Can you work these out from the model? Positions are in its coordinate system, mm. A direction names the side the tool comes from. Give positions to 0.01 mm unless a question says otherwise; leave off trailing zeros. Order: outer loops, then holes, each group sorted by start corner. A loop starts at its lowest first (then second) coordinate and runs counter-clockwise, first axis right, second up. Notation, with made-up numbers: (82, 73.25) - (99, 73.25) arc R32 ccw to (99, 110.25) - close; hole circle Ø10 at (-0.5, 81.25). An arc over 180 degrees is marked (long way). Answer as a JSON object with one key per item and string values.
```python
from build123d import *

# Parameters (mm, degrees)
SKETCH1_R           = 3.95
SKETCH1_R_2         = 1.475
SKETCH1_R_3         = 22.5
SKETCH1_R_4         = 2.4
SKETCH1_R_5         = 1.975
BOSS_EXTRUDE1_DEPTH = 5


with BuildPart() as part:
    # Sketch1 → Boss-Extrude1 (new body)
    with BuildSketch(Plane.XY):
        with BuildLine():
            Line((35, 0), (35, 162))
            ThreePointArc((35, 162), (0, 197), (-35, 162))
            Line((-35, 162), (-35, 0))
            ThreePointArc((-35, 0), (0, -35), (35, 0))
        make_face()
        Circle(SKETCH1_R, mode=Mode.SUBTRACT)
        with Locations((0, 29)):
            Circle(SKETCH1_R_2, mode=Mode.SUBTRACT)
        with Locations((0, 162)):
            Circle(SKETCH1_R_3, mode=Mode.SUBTRACT)
        with Locations((0, 133)):
            Circle(SKETCH1_R_2, mode=Mode.SUBTRACT)
        with Locations((-30, 97)):
            Circle(SKETCH1_R_2, mode=Mode.SUBTRACT)
        with Locations((30, 97)):
            Circle(SKETCH1_R_2, mode=Mode.SUBTRACT)
        with Locations((29, 0)):
            Circle(SKETCH1_R_2, mode=Mode.SUBTRACT)
        with Locations((0, -29)):
            Circle(SKETCH1_R_2, mode=Mode.SUBTRACT)
        with Locations((-29, 0)):
            Circle(SKETCH1_R_2, mode=Mode.SUBTRACT)
        with Locations((0, 12)):
            Circle(SKETCH1_R_4, mode=Mode.SUBTRACT)
        with Locations((12, 0)):
            Circle(SKETCH1_R_4, mode=Mode.SUBTRACT)
        with Locations((0, -12)):
            Circle(SKETCH1_R_4, mode=Mode.SUBTRACT)
        with Locations((-12, 0)):
            Circle(SKETCH1_R_4, mode=Mode.SUBTRACT)
        with Locations((0, 191)):
            Circle(SKETCH1_R_5, mode=Mode.SUBTRACT)
        with Locations((29, 162)):
            Circle(SKETCH1_R_5, mode=Mode.SUBTRACT)
        with Locations((-29, 162)):
            Circle(SKETCH1_R_5, mode=Mode.SUBTRACT)
        with BuildLine():
            Line((4.5, 80), (4.5, 40))
            ThreePointArc((4.5, 40), (0, 35.5), (-4.5, 40))
            Line((-4.5, 40), (-4.5, 80))
            ThreePointArc((-4.5, 80), (0, 84.5), (4.5, 80))
        make_face(mode=Mode.SUBTRACT)
        with BuildLine():
            Line((21.5, 80), (21.5, 40))
            ThreePointArc((21.5, 40), (17, 35.5), (12.5, 40))
            Line((12.5, 40), (12.5, 80))
            ThreePointArc((12.5, 80), (17, 84.5), (21.5, 80))
        make_face(mode=Mode.SUBTRACT)
        with BuildLine():
            Line((-21.5, 80), (-21.5, 40))
            ThreePointArc((-21.5, 40), (-17, 35.5), (-12.5, 40))
            Line((-12.5, 40), (-12.5, 80))
            ThreePointArc((-12.5, 80), (-17, 84.5), (-21.5, 80))
        make_face(mode=Mode.SUBTRACT)
        with BuildLine():
            Line((6.5, 121.5), (6.5, 108.5))
            ThreePointArc((6.5, 108.5), (0, 102), (-6.5, 108.5))
            Line((-6.5, 108.5), (-6.5, 121.5))
            ThreePointArc((-6.5, 121.5), (0, 128), (6.5, 121.5))
        make_face(mode=Mode.SUBTRACT)
        with BuildLine():
            Line((26.5, 120.946496324), (26.5, 107.946496324))
            ThreePointArc((26.5, 107.946496324), (20, 101.446496324), (13.5, 107.946496324))
            Line((13.5, 107.946496324), (13.5, 120.946496324))
            ThreePointArc((13.5, 120.946496324), (20, 127.446496324), (26.5, 120.946496324))
        make_face(mode=Mode.SUBTRACT)
        with BuildLine():
            Line((-26.5, 120.946496324), (-26.5, 107.946496324))
            ThreePointArc((-26.5, 107.946496324), (-20, 101.446496324), (-13.5, 107.946496324))
            Line((-13.5, 107.946496324), (-13.5, 120.946496324))
            ThreePointArc((-13.5, 120.946496324), (-20, 127.446496324), (-26.5, 120.946496324))
        make_face(mode=Mode.SUBTRACT)
    extrude(amount=BOSS_EXTRUDE1_DEPTH)


solid = part.part
```
Q1. We'd pull the mould along X, two halves only. Please class faces 1 (the face through (0.77, 196.99, 2.46)), 2 (the face through (0.1, 35.5, 2.5)), 3 (the face through (-19.857, 127.445, 2.465)), 4 (the face through (7, 83, 5)): released by +X, released by -X, zero draft, split by the parting line, or undercut.
Recorded:
{"face 1": "split by the parting line", "face 2": "undercut", "face 3": "undercut", "face 4": "zero draft"}
Q2. Which directions (+Z, -Z, +X, -X, +Y, -Y) give clear straight access to the entire face, cutting with the end or side of a thin tool? Please do faces 5 (the face through (0, 128, 2)), 6 (the face through (35, 80, 2)).
Recorded:
{"face 5": "+Z, -Z", "face 6": "+Z, -Z, +X, +Y, -Y"}
Q3. If we section it at B-B, the plane y = 146.5: Please give me the cut outline in (x, z), then the cut area to 3 significant figures.
Recorded:
{"outline": "(-35, 0) - (-16.31, 0) - (-16.31, 5) - (-35, 5) - close; (16.31, 0) - (35, 0) - (35, 5) - (16.31, 5) - close", "area": "187 mm^2"}
Q4. If we section it at A-A, the plane y = 62: Please give me the cut outline in (x, z), then the cut area to 3 significant figures.
Recorded:
{"outline": "(-35, 0) - (-21.5, 0) - (-21.5, 5) - (-35, 5) - close; (-12.5, 0) - (-4.5, 0) - (-4.5, 5) - (-12.5, 5) - close; (4.5, 0) - (12.5, 0) - (12.5, 5) - (4.5, 5) - close; (21.5, 0) - (35, 0) - (35, 5) - (21.5, 5) - close", "area": "215 mm^2"}
Q5. I'm going to push a flat-ended pin straight in: pin 1 Ø2 at (x, z) = (4.5, 2.5) entering from -Y. Where does the tip first touch, or does it pass through?
Recorded:
{"pin 1": "stops at y = -34.82"}
Q6. If we section it at C-C, the plane y = 111.5: Please give me the cut outline in (x, z), then the cut area to 3 significant figures.
Recorded:
{"outline": "(-35, 0) - (-26.5, 0) - (-26.5, 5) - (-35, 5) - close; (-13.5, 0) - (-6.5, 0) - (-6.5, 5) - (-13.5, 5) - close; (6.5, 0) - (13.5, 0) - (13.5, 5) - (6.5, 5) - close; (26.5, 0) - (35, 0) - (35, 5) - (26.5, 5) - close", "area": "155 mm^2"}
Q7. I need wall thicknesses on L1, parallel to X at y = 69, z = 1.25; L2, parallel to X at y = 97, z = 3.35 (3 decimals); L3, parallel to Y at x = -30, z = 1.35 (3 decimals). Which ranges of each line are inside material? Lowest first, please.
Recorded:
{"L1": "x = -35 to -21.5, -12.5 to -4.5, 4.5 to 12.5, 21.5 to 35", "L2": "x = -35 to -31.475, -28.525 to 28.525, 31.475 to 35", "L3": "y = -18.028 to -1.084, 1.084 to 95.525, 98.475 to 160.297, 163.703 to 180.028"}
Q8. If we section it at D-D, the plane z = 0.9: Count the separate pieces of the cut face and the enclosed holes in it, then the cut area to 3 significant figures.
Recorded:
{"separate pieces": "1", "enclosed holes": "22", "area": "11,200 mm^2"}
